Could you check a few things on this model? Use its own coordinates, in mm. A direction names the side the tool comes from. Coordinates: 2 decimals unless noted, no trailing zeros. Order: outer loops, then holes, each group sorted by start corner. A loop starts at its lowest first (then second) coordinate and runs counter-clockwise, first axis right, second up. Notation, with made-up numbers: (-32, 82.5) -> (7, 82.5) arc R26 ccw to (7, 116.5) -> close; hole circle Ø8 at (21.5, 35). An arc over 180 degrees is marked (long way). Use a Markdown table: item, result. Add a question column.
1) If we section it at A-A (x = 0): Write out the boundary of the cut face in (y, z).
2) If we section it at B-B (x = -13): Write out the boundary of the cut face in (y, z), plus the area to 3 significant figures.
3) Which directions (+Z, -Z, +X, -X, +Y, -Y) give clear straight access to the entire face, cutting with the end or side of a thin tool? Please do faces 4 (the cylindrical face through (40.681, 22.713, -3.219)), 5 (the flat face through (-50.8, 29, -3)).
4) If we section it at D-D (y = 38.5): Write out the boundary of the cut face in (x, z).
5) If I drill on L1, parallel to Y at x = 0, z = -2; L2, parallel to Y at x = 41.5, z = -2.25; L3, parallel to X at y = 8.5, z = -1.5, over which ranges is the centre line in solid material (lowest first)? Write a range as [from, to].
6) Thinking about a two-plate mould opening in X: for faces 1 (the flat face through (50.8, 28, -3)), 2 (the flat face through (-1, 0, -3)), 3 (the cylindrical face through (-32.836, 89.059, -3.219)), which applies, +X half, -X half, draft (parallel to the pull), parting line (faces both ways), or undercut?
7) If we section it at C-C (z = -3.5): Give the number of separate pieces and of enclosed holes in the cut face, plus the area to 3 significant figures.
```python
from build123d import *

# Parameters (mm, degrees)
SKETCH1_R                = 44.958
BOSS_EXTRUDE1_DEPTH      = 6.35
M3_CLEARANCE_HOLE2_D     = 3.4
M3_CLEARANCE_HOLE2_DEPTH = 25.4
M3_CLEARANCE_HOLE2_TIP   = 1.021463052
M3_CLEARANCE_HOLE3_D     = 3.7
M3_CLEARANCE_HOLE3_DEPTH = 25.4
M3_CLEARANCE_HOLE3_TIP   = 1.111592145
CUT_EXTRUDE1_START       = -6.35
CUT_EXTRUDE1_DEPTH       = 6.35


# Read off the part's stored shape, not the designer's step: Cut-Extrude1
with BuildPart() as part:
    # Sketch1 → Boss-Extrude1 (new body)
    with BuildSketch(Plane.XY):
        with BuildLine():
            Line((50.8, 0), (50.8, 56.896))
            ThreePointArc((50.8, 56.896), (0, 107.696), (-50.8, 56.896))
            Line((-50.8, 56.896), (-50.8, 0))
            Line((-50.8, 0), (50.8, 0))
        make_face()
        with Locations((0, 56.896)):
            Circle(SKETCH1_R, mode=Mode.SUBTRACT)
    extrude(amount=-BOSS_EXTRUDE1_DEPTH)

    # M3 Clearance Hole2
    with Locations(Plane.XY):
        with Locations((-36.83, 10.7442)):
            Hole(M3_CLEARANCE_HOLE2_D / 2, depth=M3_CLEARANCE_HOLE2_DEPTH)
            with Locations((0, 0, -(M3_CLEARANCE_HOLE2_DEPTH + M3_CLEARANCE_HOLE2_TIP / 2))):  # 118° drill point
                Cone(0, M3_CLEARANCE_HOLE2_D / 2, M3_CLEARANCE_HOLE2_TIP, mode=Mode.SUBTRACT)

    # M3 Clearance Hole3
    with Locations(Plane.XY):
        with Locations((0, 104.394), (34.304578382, 90.184578382), (34.304578383, 21.575421618), (0, 7.366), (-34.304578382, 21.575421618), (-34.304578382, 90.184578382)):
            Hole(M3_CLEARANCE_HOLE3_D / 2, depth=M3_CLEARANCE_HOLE3_DEPTH)
            with Locations((0, 0, -(M3_CLEARANCE_HOLE3_DEPTH + M3_CLEARANCE_HOLE3_TIP / 2))):  # 118° drill point
                Cone(0, M3_CLEARANCE_HOLE3_D / 2, M3_CLEARANCE_HOLE3_TIP, mode=Mode.SUBTRACT)

    # Cut-Extrude1 outline → Cut-Extrude1 (cut)
    with BuildSketch(Plane.XY.offset(CUT_EXTRUDE1_START)):
        with BuildLine():
            Line((42.49, 9.398), (42.525, 20.828))
            ThreePointArc((42.525, 20.828), (40.64, 22.713), (38.755, 20.828))
            Line((38.755, 20.828), (38.79, 9.398))
            ThreePointArc((38.79, 9.398), (40.64, 7.548), (42.49, 9.398))
        make_face()
    extrude(amount=CUT_EXTRUDE1_DEPTH, mode=Mode.SUBTRACT)


solid = part.part
```
Answer sheet:
| question | item | result |
|---|---|---|
| 1 | outline | (0, -6.35) -> (5.52, -6.35) -> (5.52, 0) -> (0, 0) -> close; (9.22, -6.35) -> (11.94, -6.35) -> (11.94, 0) -> (9.22, 0) -> close; (101.85, -6.35) -> (102.54, -6.35) -> (102.54, 0) -> (101.85, 0) -> close; (106.24, -6.35) -> (107.7, -6.35) -> (107.7, 0) -> (106.24, 0) -> close |
| 2 | outline | (0, -6.35) -> (13.86, -6.35) -> (13.86, 0) -> (0, 0) -> close; (99.93, -6.35) -> (106, -6.35) -> (106, 0) -> (99.93, 0) -> close |
| 2 | area | 127 mm2 |
| 3 | face 4 | +Z, -Z |
| 3 | face 5 | +Z, -Z, -X, +Y, -Y |
| 4 | outline | (-50.8, -6.35) -> (-41.02, -6.35) -> (-41.02, 0) -> (-50.8, 0) -> close; (41.02, -6.35) -> (50.8, -6.35) -> (50.8, 0) -> (41.02, 0) -> close |
| 5 | L1 | [0, 5.52], [9.22, 11.94], [101.85, 102.54], [106.24, 107.7] |
| 5 | L2 | [0, 7.76], [22.51, 39.61], [74.19, 86.19] |
| 5 | L3 | [-50.8, -1.46], [1.46, 39.02], [42.26, 50.8] |
| 6 | face 1 | +X half |
| 6 | face 2 | draft |
| 6 | face 3 | undercut |
| 7 | separate pieces | 1 |
| 7 | enclosed holes | 9 |
| 7 | area | 3,360 mm2 |
